Source: CAD feature listing. Evaluate the final solid. Frame: model axes, mm. Face numbers are marked on the shaded views. A direction names the side the tool comes from. Round coordinates to 2 decimals unless told otherwise and drop trailing zeros. Loops run counter-clockwise (first coordinate to the right, second up) from the corner with the lowest first, then second, coordinate; pieces in that order, holes last. Notation, with made-up numbers: M 38,24.5 L 81,24.5 A22 cw 81,54.5 Z; hole C 89,55.25 d11. An arc over 180 degrees is marked long. Answer as a JSON object with one key per item and string values.
from build123d import *


with BuildPart() as part:
    # Sketch1 → Revolve1 (revolve)
    with BuildSketch(Plane.XY, mode=Mode.PRIVATE) as revolve1_sk:
        Polygon((11.5, 150), (11.5, 114.942528736), (51.5, 0), (51.5, 9.127775749), (14.5, 115.44961483), (14.5, 147), (24.5, 147), (24.5, 150), (14.5, 150), align=None)
    revolve(revolve1_sk.sketch.rotate(Axis((0, 0, 0), (0, 1, 0)), 90), axis=Axis((0, 0, 0), (0, 1, 0)))  # turned: the seam where the file's is


solid = part.part
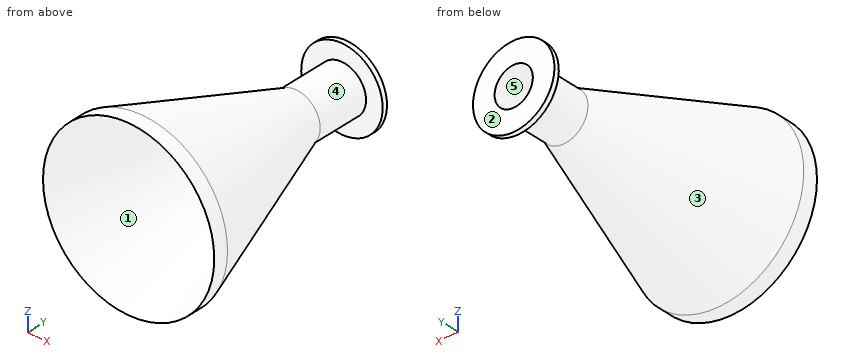
Item 1: Pull-direction query (X, two-part tool) for the marked faces 1, 2 and 3; classes: pulls with the +X half, pulls with the -X half, needs draft (parallel to the pull), parting line crosses it, or undercut.
Answer sheet:
{"face 1": "undercut", "face 2": "needs draft", "face 3": "parting line crosses it"}
Item 2: Section C-C on y = 138. Return the cut outline in (x, z).
Answer sheet:
{"outline": "C 0,0 d29; hole C 0,0 d23"}
Item 3: Section A-A on z = 0. Return the cut outline in (x, y).
Answer sheet:
{"outline": "M -51.5,0 L -11.5,114.94 L -11.5,150 L -24.5,150 L -24.5,147 L -14.5,147 L -14.5,115.45 L -51.5,9.13 Z; M 11.5,114.94 L 51.5,0 L 51.5,9.13 L 14.5,115.45 L 14.5,147 L 24.5,147 L 24.5,150 L 11.5,150 Z"}
Item 4: Contact query for flat-ended pins moving along their axis: pin 1 Ø1.5 at (x, y) = (-4.5, 83.5) entering from +Z; pin 2 Ø1 at (y, z) = (51, 11.5) entering from -X; pin 3 Ø5 at (y, z) = (75.5, -11.5) entering from +X. Output: stop coordinate, or through.
Answer sheet:
{"pin 1": "stops at z = 25.51", "pin 2": "stops at x = -35.34", "pin 3": "stops at x = 27.34"}
Item 5: Line query: probe 1 along X at (y, z) = (130, 0); probe 2 along X at (y, z) = (55, 14); probe 3 along Z at (x, y) = (14, 8.5). Output: solid intervals per line, ascending. Write a range as from..to.
Answer sheet:
{"probe 1": "x = -14.5..-11.5, 11.5..14.5", "probe 2": "x = -32.66..-29.17, 29.17..32.66", "probe 3": "z = -49.56..-46.48, 46.48..49.56"}
Item 6: Section D-D on y = 41. Return the cut outline in (x, z).
Answer sheet:
{"outline": "C 0,0 d80.82; hole C 0,0 d74.46"}
Item 7: Section B-B on x = 0. Return the cut outline in (y, z).
Answer sheet:
{"outline": "M 0,-51.5 L 9.13,-51.5 L 115.45,-14.5 L 147,-14.5 L 147,-24.5 L 150,-24.5 L 150,-11.5 L 114.94,-11.5 Z; M 0,51.5 L 114.94,11.5 L 150,11.5 L 150,24.5 L 147,24.5 L 147,14.5 L 115.45,14.5 L 9.13,51.5 Z"}
Item 8: Access query for the marked faces 4 and 5. Directions: +Z, -Z, +X, -X, +Y, -Y. A direction counts if a zero-diameter tool reaches every point of the face in a straight line with its end or side. Return the directions, or none.
Answer sheet:
{"face 4": "none", "face 5": "+Y, -Y"}
